Model file for the job. Use its own axes, mm. Face numbers are marked on the shaded views. A direction names the side the tool comes from. Give positions to 0.01 mm unless a question says otherwise; leave off trailing zeros. Write each loop counter-clockwise with the first axis right and the second up, starting at its lowest first coordinate (ties: lowest second). Pieces come first, ordered by that corner, then holes. Notation, with made-up numbers: M 20.5,-38.75 L 59.5,-38.75 A25 ccw 59.5,-21.75 Z; hole C 3,-5 d3. An arc over 180 degrees is marked long. Answer as a JSON object with one key per item and string values. Group by question number.
```python
from build123d import *

# Parameters (mm, degrees)
SKETCH1_W                  = 20
SKETCH1_H                  = 30
BOSS_EXTRUDE1_DEPTH        = 3
F_3_4_3_4_DIAMETER_HOLE1_D = 3.4
SKETCH5_R                  = 3.4
CUT_EXTRUDE1_DEPTH         = 0.5
FILLET1_R                  = 3
SKETCH7_W                  = 8
SKETCH7_H                  = 15
BOSS_EXTRUDE3_DEPTH        = 11
CUT_EXTRUDE3_DEPTH         = 25.839484697
CUT_EXTRUDE3_DEPTH_BACK    = 25.839484697
SKETCH11_OUTSIDE_W         = 29.736
SKETCH11_OUTSIDE_H         = 39.736
SKETCH11_OUTSIDE_R         = 2.5
CUT_EXTRUDE4_DEPTH         = 22.118712082
SKETCH12_W                 = 7.43023475
SKETCH12_H                 = 21.108621448
CUT_EXTRUDE5_DEPTH         = 29.653097564
SKETCH13_R                 = 3.4
SKETCH13_R_2               = 2.75
BOSS_EXTRUDE4_DEPTH        = 0.5
SKETCH14_W                 = 15
SKETCH14_H                 = 15
BOSS_EXTRUDE5_DEPTH        = 5
FILLET2_R                  = 3


with BuildPart() as part:
    # Sketch1 → Boss-Extrude1 (new body)
    with BuildSketch(Plane.XY):
        Rectangle(SKETCH1_W, SKETCH1_H)
    extrude(amount=BOSS_EXTRUDE1_DEPTH)

    # Ø3.4 (3.4) Diameter Hole1 (through all)
    with Locations(Plane.XY.offset(3)):
        with Locations((-6.5, 11.5), (6.5, 11.5), (6.5, -11.5), (-6.5, -11.5)):
            Hole(F_3_4_3_4_DIAMETER_HOLE1_D / 2)

    # Sketch5 → Cut-Extrude1 (cut)
    with BuildSketch(Plane(origin=(0, 0, 0), x_dir=(-1, 0, 0), z_dir=(0, 0, -1))):
        Circle(SKETCH5_R)
    extrude(amount=-CUT_EXTRUDE1_DEPTH, mode=Mode.SUBTRACT)

    # Fillet1
    fillet1_edges = [part.edges().sort_by_distance(p)[0] for p in [
        (10, -15, 1.5),
        (-10, -15, 1.5),
        (-10, 15, 1.5),
        (10, 15, 1.5),
    ]]
    fillet(fillet1_edges, radius=FILLET1_R)

    # Sketch7 → Boss-Extrude3 (add)
    with BuildSketch(Plane.XY.offset(3)):
        Rectangle(SKETCH7_W, SKETCH7_H)
    extrude(amount=BOSS_EXTRUDE3_DEPTH)

    # Sketch8 → Cut-Extrude3 (cut, two sides: drawn at the far end of the back side and taken through both)
    with BuildSketch(Plane(origin=(4, 0, 0), x_dir=(0, 0, -1), z_dir=(1, 0, 0)).offset(-CUT_EXTRUDE3_DEPTH_BACK)):
        Polygon((-14, -6), (-14, -7), (-13.133974596, -6.5), align=None)
        Polygon((-13.133974596, -7.5), (-14, -7), (-14, -7.5), align=None)
        Polygon((-14, -5), (-14, -6), (-13.133974596, -5.5), align=None)
        Polygon((-14, -4), (-14, -5), (-13.133974596, -4.5), align=None)
        Polygon((-14, -3), (-14, -4), (-13.133974596, -3.5), align=None)
        Polygon((-14, 7), (-13.133974596, 7.5), (-14, 7.5), align=None)
        Polygon((-14, -2), (-14, -3), (-13.133974596, -2.5), align=None)
        Polygon((-13.133974596, 6.5), (-14, 7), (-14, 6), align=None)
        Polygon((-14, -1), (-14, -2), (-13.133974596, -1.5), align=None)
        Polygon((-13.133974596, 5.5), (-14, 6), (-14, 5), align=None)
        Polygon((-14, 0), (-14, -1), (-13.133974596, -0.5), align=None)
        Polygon((-13.133974596, 4.5), (-14, 5), (-14, 4), align=None)
        Polygon((-14, 1), (-14, 0), (-13.133974596, 0.5), align=None)
        Polygon((-13.133974596, 3.5), (-14, 4), (-14, 3), align=None)
        Polygon((-14, 2), (-14, 1), (-13.133974596, 1.5), align=None)
        Polygon((-13.133974596, 2.5), (-14, 3), (-14, 2), align=None)
    extrude(amount=CUT_EXTRUDE3_DEPTH + CUT_EXTRUDE3_DEPTH_BACK, mode=Mode.SUBTRACT)

    # Sketch11 outside → Cut-Extrude4 (cut, through all)
    with BuildSketch(Plane.XY.offset(3)):
        Rectangle(SKETCH11_OUTSIDE_W, SKETCH11_OUTSIDE_H)
        Circle(SKETCH11_OUTSIDE_R, mode=Mode.SUBTRACT)
    extrude(amount=CUT_EXTRUDE4_DEPTH, mode=Mode.SUBTRACT)

    # Sketch12 → Cut-Extrude5 (cut, through all)
    with BuildSketch(Plane(origin=(10, 0, 0), x_dir=(0, 0, -1), z_dir=(1, 0, 0))):
        with Locations((-11.715117375, -0.112579314)):
            Rectangle(SKETCH12_W, SKETCH12_H)
    extrude(amount=-CUT_EXTRUDE5_DEPTH, mode=Mode.SUBTRACT)

    # Sketch13 → Boss-Extrude4 (add)
    with BuildSketch(Plane(origin=(0, 0, 0), x_dir=(-1, 0, 0), z_dir=(0, 0, -1))):
        Circle(SKETCH13_R)
        Circle(SKETCH13_R_2, mode=Mode.SUBTRACT)
    extrude(amount=-BOSS_EXTRUDE4_DEPTH)

    # Sketch14 → Boss-Extrude5 (add)
    with BuildSketch(Plane.XY.offset(3)):
        Rectangle(SKETCH14_W, SKETCH14_H)
    extrude(amount=BOSS_EXTRUDE5_DEPTH)

    # Fillet2
    fillet2_edges = [part.edges().sort_by_distance(p)[0] for p in [
        (7.5, 7.5, 5.5),
        (7.5, -7.5, 5.5),
        (-7.5, -7.5, 5.5),
        (-7.5, 7.5, 5.5),
    ]]
    fillet(fillet2_edges, radius=FILLET2_R)


solid = part.part
```
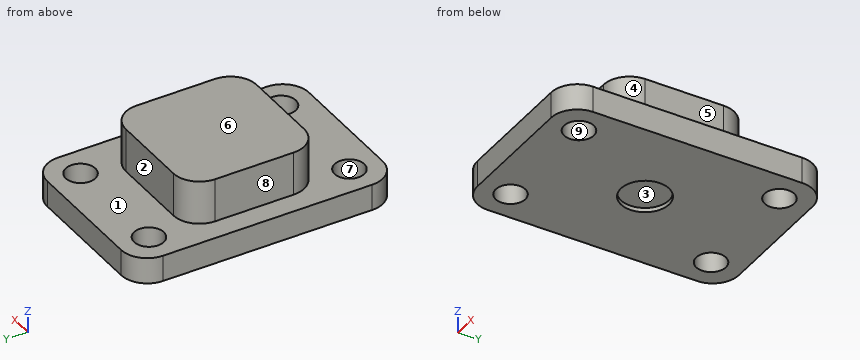
Q1. Slice it at D-D, the plane z = 4.25. Write the cut outline in (x, y), then the cut area to 3 significant figures.
Q2. Slice it at C-C, the plane x = 5.5. Write the cut outline in (y, z), then the cut area to 3 significant figures.
Q3. Wall check: L1, parallel to Y at x = -6.5, z = 2.45; L2, parallel to Y at x = 7.75, z = 1.25; L3, parallel to Y at x = 4, z = 4. Give the ranges that are in metal, low to high.
Q4. Two-plate mould, pull along X, no slides. Class the marked faces 6, 7, 8 and 9: +X half, -X half, draft (parallel to the pull), parting line (faces both ways), or undercut.
Q5. 3-axis set-ups, long thin cutter, end or side, ignore diameter. For the marked faces 1, 2, 3, 4 and 5: which of +Z, -Z, +X, -X, +Y, -Y reach the whole face in a straight line?
Q6. Slice it at B-B, the plane z = 2.5. Write the cut outline in (x, y).
Q7. Drop flat-ended pins along their axis: P1, Ø2.5, axis at y = 1.5, z = 5, coming from the -X side; P2, Ø1.6, axis at x = 1.5, y = 0, coming from the -Z side; P3, Ø2.5, axis at x = -2, z = 6.5, coming from the -Y side. Give the stop position or say it passes through.
Q8. Slice it at A-A, the plane y = 11.5. Write the cut outline in (x, z).
Solved:
{
 "1": {"outline": "M -7.5,-4.5 A3 ccw -4.5,-7.5 L 4.5,-7.5 A3 ccw 7.5,-4.5 L 7.5,4.5 A3 ccw 4.5,7.5 L -4.5,7.5 A3 ccw -7.5,4.5 Z", "area": "217 mm²"},
 "2": {"outline": "M -15,0 L -12.87,0 L -12.87,3 L -15,3 Z; M -10.13,0 L 10.13,0 L 10.13,3 L 7.33,3 L 7.33,8 L -7.33,8 L -7.33,3 L -10.13,3 Z; M 12.87,0 L 15,0 L 15,3 L 12.87,3 Z", "area": "147 mm²"},
 "3": {"L1": "y = -15 to -13.2, -9.8 to 9.8, 13.2 to 15", "L2": "y = -14.9 to -12.65, -10.35 to 10.35, 12.65 to 14.9", "L3": "y = -7.5 to 7.5"},
 "4": {"face 6": "draft", "face 7": "undercut", "face 8": "-X half", "face 9": "undercut"},
 "5": {"face 1": "+Z", "face 2": "+Z, +X, -X, +Y", "face 3": "-Z", "face 4": "+Z, +X, -Y", "face 5": "+Z, +X, +Y, -Y"},
 "6": {"outline": "M -10,-12 A3 ccw -7,-15 L 7,-15 A3 ccw 10,-12 L 10,12 A3 ccw 7,15 L -7,15 A3 ccw -10,12 Z; hole C -6.5,-11.5 d3.4; hole C -6.5,11.5 d3.4; hole C 6.5,-11.5 d3.4; hole C 6.5,11.5 d3.4"},
 "7": {"P1": "stops at x = -7.5", "P2": "stops at z = 0.5", "P3": "stops at y = -7.5"},
 "8": {"outline": "M -10,0 L -8.2,0 L -8.2,3 L -10,3 Z; M -4.8,0 L 4.8,0 L 4.8,3 L -4.8,3 Z; M 8.2,0 L 10,0 L 10,3 L 8.2,3 Z"}
}
